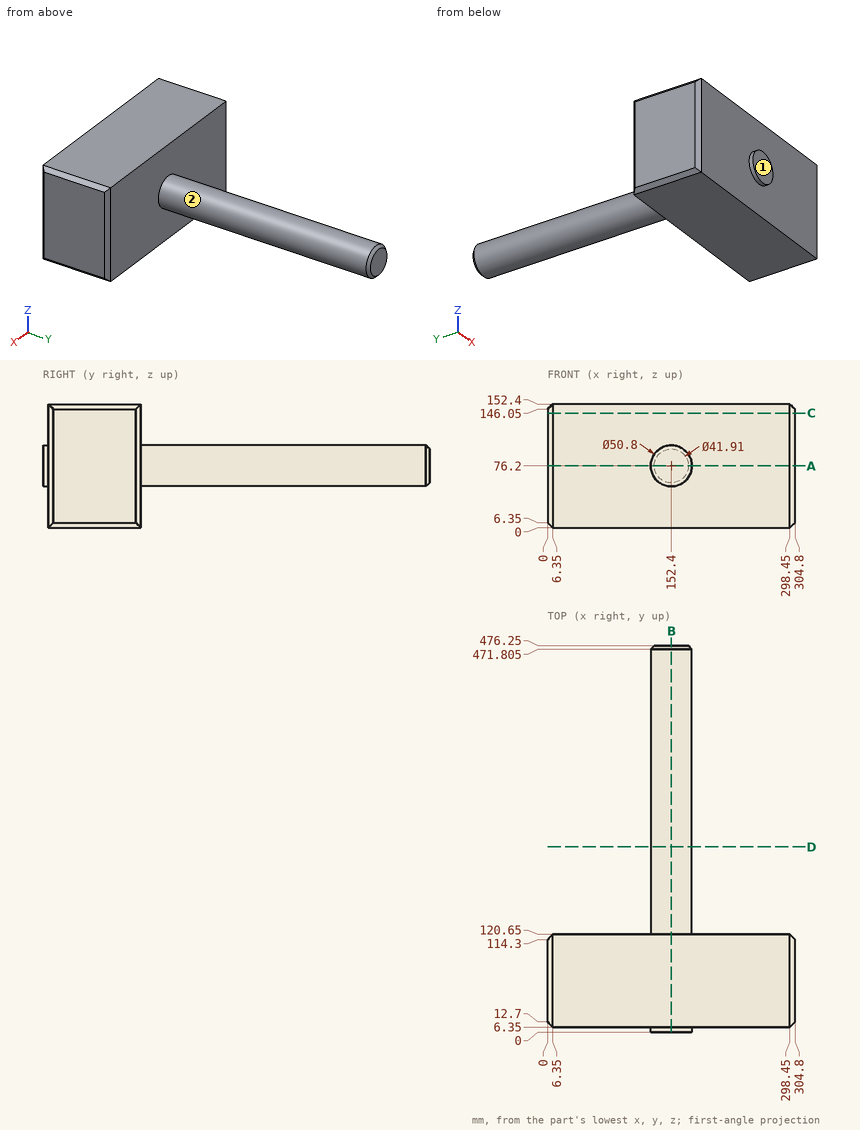
Print and shaded views of the part. All mm, measured from the part's lowest x, y and z. A direction names the side the tool comes from. Give positions to 0.01 mm unless a question says otherwise; leave off trailing zeros. Loops run counter-clockwise (first coordinate to the right, second up) from the corner with the lowest first, then second, coordinate; pieces in that order, holes last. Notation, with made-up numbers: (-15.5, 44) -> (10.5, 44) arc R14 cw to (10.5, 56) -> close; hole circle Ø8 at (-33.75, 63). An arc over 180 degrees is marked (long way). Use CSV: the item, a comma, the result in double quotes. Start each with the question number.
1) Slice it at A-A on z = 76.2. Give the cut face in (x, y) (3 decimals).
2) Flat gauge pins, fed straight in: pin 1 Ø10 at (x, z) = (223, 117) entering from -Y; pin 2 Ø8 at (x, y) = (166.5, 308) entering from +Z; pin 3 Ø8 at (y, z) = (250.5, 62) entering from +X. Where does each tip first touch, or does it go through?
3) Slice it at B-B on x = 152.4. Give the cut face in (y, z) (3 decimals), plus the area to 3 significant figures.
4) Wall check: line 1 (Y direction, x = 47, z = 94); line 2 (X direction, y = 278, z = 96.5); line 3 (X direction, y = 246.5, z = 71.5). Give the ranges that are in metal, low to high.
5) Tool access for the marked faces 1 and 2: list every direction of +Z, -Z, +X, -X, +Y, -Y with a clear straight run to the whole face (end or side of a thin tool).
6) Slice it at C-C on z = 141. Give the cut face in (x, y).
7) Slice it at D-D on y = 228.5. Give the cut face in (x, z).
Computed values:
1,outline,"(0, 12.7) -> (6.35, 6.35) -> (127, 6.35) -> (127, 0) -> (177.8, 0) -> (177.8, 6.35) -> (298.45, 6.35) -> (304.8, 12.7) -> (304.8, 114.3) -> (298.45, 120.65) -> (177.8, 120.65) -> (177.8, 471.805) -> (173.355, 476.25) -> (131.445, 476.25) -> (127, 471.805) -> (127, 120.65) -> (6.35, 120.65) -> (0, 114.3) -> close"
2,pin 1,"stops at y = 6.35"
2,pin 2,"stops at z = 99.51"
2,pin 3,"stops at x = 175.66"
3,outline,"(0, 50.8) -> (6.35, 50.8) -> (6.35, 0) -> (120.65, 0) -> (120.65, 50.8) -> (471.805, 50.8) -> (476.25, 55.245) -> (476.25, 97.155) -> (471.805, 101.6) -> (120.65, 101.6) -> (120.65, 152.4) -> (6.35, 152.4) -> (6.35, 101.6) -> (0, 101.6) -> close"
3,area,"35,800 mm^2"
4,line 1,"y = 6.35 to 120.65"
4,line 2,"x = 137.13 to 167.67"
4,line 3,"x = 127.44 to 177.36"
5,face 1,"+Z, -Z, +X, -X, -Y"
5,face 2,"+Y"
6,outline,"(0, 12.7) -> (6.35, 6.35) -> (298.45, 6.35) -> (304.8, 12.7) -> (304.8, 114.3) -> (298.45, 120.65) -> (6.35, 120.65) -> (0, 114.3) -> close"
7,outline,"circle Ø50.8 at (152.4, 76.2)"
